Can you work these out from the model? Positions are in its coordinate system, mm. A direction names the side the tool comes from. Round coordinates to 2 decimals unless told otherwise and drop trailing zeros. Order: outer loops, then holes, each group sorted by start corner. A loop starts at its lowest first (then second) coordinate and runs counter-clockwise, first axis right, second up.
Q1. If we section it at C-C (y = 1): Please give me the cut outline in (x, z).
Q2. We'd pull the mould along X, two halves only. Please class faces 1 (the face through (-3, 5, 44.45)), 2 (the face through (-3, 22, 584.2)), 3 (the face through (-78.359, 5, 288)), 4 (the face through (32.1, 24, 54.4)): pulls with the +X half, pulls with the -X half, needs draft (parallel to the pull), parting line crosses it, or undercut.
Q3. If we section it at A-A (x = -18): Please give me the cut outline in (y, z).
Q4. If I drill on line 1 (Z direction, x = 0, y = 19); line 2 (Z direction, x = 0, y = -3.5); line 3 (Y direction, x = 48, z = 320), over which ranges is the centre line in solid material (lowest first)?
Q5. If we section it at B-B (z = 25.4): Please give me the cut outline in (x, y), plus the area to 3 significant figures.
Q6. Will this pin go through, and if not, where does the flat tip stop? P1, Ø7.5, axis at x = -2, y = 7.5, coming from the +Z side.
Q7. For faces 5 (the face through (-45, 17.692, 318)), 6 (the face through (-2, 24, 571.5)), 7 (the face through (74.041, 5, 288)), which set-ups out of +Z, -Z, +X, -X, +Y, -Y let a thin tool reach every point of the face, with its end or its side?
Q8. If we section it at D-D (z = 258.5): Please give me the cut outline in (x, y).
from build123d import *

# Parameters (mm, degrees)
F0_W     = 152.4
F0_H     = 50.8
F1_DEPTH = 584.2
F2_R     = 12.7
F3_DEPTH = 50.801
F4_W     = 76.2
F4_H     = 520.7
F5_DEPTH = 25.4
F6_R     = 12.7
F7_W     = 127
F7_H     = 25.4
F8_DEPTH = 539.75


with BuildPart() as f1:
    # F0 (on Top) → F1 (new body)
    with BuildSketch(Plane.XY):
        with Locations((-2.158545, 4.991524)):
            Rectangle(F0_W, F0_H)
    extrude(amount=F1_DEPTH)

    # F2 (on face) → F3 (cut, through all)
    with BuildSketch(Plane.XZ.offset(20.408476)):
        with Locations((0, 25.4)):
            Circle(F2_R)
    extrude(amount=-F3_DEPTH, mode=Mode.SUBTRACT)

    # F4 (on face) → F5 (cut)
    with BuildSketch(Plane(origin=(0, 30.391524, 0), x_dir=(-1, 0, 0), z_dir=(0, 1, 0))):
        with Locations((2.158545, 311.15)):
            Rectangle(F4_W, F4_H)
    extrude(amount=-F5_DEPTH, mode=Mode.SUBTRACT)

    # F6
    f6_edges = [f1.edges().sort_by_distance(p)[0] for p in [
        (35.941455, 17.691524, 50.8),
        (-40.258545, 17.691524, 50.8),
        (-40.258545, 17.691524, 571.5),
        (35.941455, 17.691524, 571.5),
    ]]
    fillet(f6_edges, radius=F6_R)

    # F7 (on face) → F8 (cut)
    with BuildSketch(Plane.XY.offset(584.2)):
        with Locations((-2.158545, 4.991524)):
            Rectangle(F7_W, F7_H)
    extrude(amount=-F8_DEPTH, mode=Mode.SUBTRACT)


solid = f1.part
Solution:
1. outline: (-78.36, 0) - (74.04, 0) - (74.04, 584.2) - (61.34, 584.2) - (61.34, 44.45) - (-65.66, 44.45) - (-65.66, 584.2) - (-78.36, 584.2) - close; hole circle Ø25.4 at (0, 25.4)
2. face 1: undercut
2. face 2: needs draft
2. face 3: pulls with the -X half
2. face 4: undercut
3. outline: (-20.41, 0) - (30.39, 0) - (30.39, 50.8) - (17.69, 50.8) - (17.69, 44.45) - (-7.71, 44.45) - (-7.71, 584.2) - (-20.41, 584.2) - close; (17.69, 571.5) - (30.39, 571.5) - (30.39, 584.2) - (17.69, 584.2) - close
4. line 1: z = 0 to 12.7, 38.1 to 50.8, 571.5 to 584.2
4. line 2: z = 0 to 12.7, 38.1 to 44.45
4. line 3: y = -20.41 to -7.71, 17.69 to 30.39
5. outline: (-78.36, -20.41) - (-12.7, -20.41) - (-12.7, 30.39) - (-78.36, 30.39) - close; (12.7, -20.41) - (74.04, -20.41) - (74.04, 30.39) - (12.7, 30.39) - close
5. area: 6,450 mm2
6. P1: stops at z = 44.45
7. face 5: +Z
7. face 6: +Y
7. face 7: +Z, -Z, +X, +Y, -Y
8. outline: (-78.36, -20.41) - (74.04, -20.41) - (74.04, 30.39) - (35.94, 30.39) - (35.94, 17.69) - (61.34, 17.69) - (61.34, -7.71) - (-65.66, -7.71) - (-65.66, 17.69) - (-40.26, 17.69) - (-40.26, 30.39) - (-78.36, 30.39) - close
